Design review of the part built by this model. Coordinates are the model's own, in mm. A direction names the side the tool comes from. Round coordinates to 2 decimals unless told otherwise and drop trailing zeros. Order: outer loops, then holes, each group sorted by start corner. A loop starts at its lowest first (then second) coordinate and runs counter-clockwise, first axis right, second up. Notation, with made-up numbers: (75, -37) - (115, -37) arc R17 cw to (115, -19) - close; hole circle Ø11 at (-20, 64.25). An arc over 180 degrees is marked (long way). Use CSV: the item, a comma, the result in double quotes.
Autodesk Inventor part; units mm, degrees
ref_plane "YZ Plane" through (0, 0, 0) normal (1, 0, 0) x (0, 1, 0)
ref_plane "XZ Plane" through (0, 0, 0) normal (0, 1, 0) x (-1, 0, 0)
ref_plane "XY Plane" through (0, 0, 0) normal (0, 0, 1) x (1, 0, 0)
sketch "Sketch1" plane through (0, 0, 0) normal (1, 0, 0) x (0, 1, 0)
  line L0 (-25.5, 21) -> (25.5, 21)
  line L1 (25.5, 21) -> (25.5, -21)
  line L2 (25.5, -21) -> (-25.5, -21)
  line L3 (-25.5, -21) -> (-25.5, 21)
  line L4 (-25.5, 21) -> (25.5, -21) construction
  line L5 (25.5, 21) -> (-25.5, -21) construction
  circle A0 centre (15.5, 16) radius 1.6
  circle A1 centre (15.5, -16) radius 1.6
  circle A2 centre (-19.5, -16) radius 1.6
  circle A3 centre (-19.5, 16) radius 1.6
  line L6 (17.5, 0) -> (-17.5, 0) construction
  line L7 (17.5, 4) -> (-17.5, 4)
  line L8 (-17.5, -4) -> (17.5, -4)
  arc A4 (17.5, -4) -> (17.5, 4) centre (17.5, 0) ccw
  arc A5 (-17.5, 4) -> (-17.5, -4) centre (-17.5, 0) ccw
  point P0 (0, 0)
  point P1 (-9.5, -16)
  point P2 (0, 0)
  point P3 (15.5, -48)
  point P4 (-19.5, -35.5845)
  dimension "d0" = 42
  dimension "d1" = 51
  dimension "d2" = 5
  dimension "d3" = 10
  dimension "d5" = 35
  dimension "d6" = 5
  dimension "d7" = 3.2
  dimension "d8" = 3.2
  dimension "d9" = 3.2
  dimension "d10" = 3.2
  dimension "d15" = 0
  dimension "d16" = 0
  dimension "d17" = 32
  dimension "d18" = 0
  dimension "d19" = 0
  dimension "d20" = 8
  dimension "d21" = 8
  dimension "d22" = 8
  dimension "d31" = 32
extrude "Extrusion1" add sketch "Sketch1" along normal blind 5
fillet "Fillet1" radius 2 4 edges at (2.5, 25.5, 21) (2.5, -25.5, 21) (2.5, -25.5, -21) (2.5, 25.5, -21)
sketch "Sketch2" plane through (0, 25.5, 19) normal (0, 1, 0) x (1, 0, 0)
  line L0 (0, 38) -> (0, 0)
  point P0 (0, 19)
  point P1 (2.5, 19)
  dimension "d23" = 2.5
hole "Hole1" at (2.5, 25.5, 0) direction (0, -1, 0) diameter 3 depth 80.45
properties part number "2mm_double_for_pulley" material "アルミニウム 6061"
1) For faces 5 (the face through (2, 0, -4)), 6 (the face through (2.54, -24.9, 20.43)), list the 3-axis set-ups (+Z, -Z, +X, -X, +Y, -Y) from which the entire face can be reached by the end or side of a thin tool; tool diameter is ignored.
Data:
face 5,"+X, -X"
face 6,"+Z, +X, -X, -Y"
2) The part is to be moulded in two halves that separate along X. For faces 1 (the face through (2, 0, 4)), 2 (the face through (0, 0, 5)), 3 (the face through (2.43, 23.32, -1.5)), 4 (the face through (2.05, -23.38, 1.43)), say which applies: +X half, -X half, draft (parallel to the pull), parting line (faces both ways), or undercut.
Data:
face 1,"draft"
face 2,"-X half"
face 3,"undercut"
face 4,"undercut"
3) We need section C-C (y = 15.5). Give the boundary of the cut face in (x, z).
Data:
outline,"(0, -21) - (5, -21) - (5, -17.6) - (0, -17.6) - close; (0, -14.4) - (5, -14.4) - (5, -4) - (0, -4) - close; (0, 4) - (5, 4) - (5, 14.4) - (0, 14.4) - close; (0, 17.6) - (5, 17.6) - (5, 21) - (0, 21) - close"
4) We need section D-D (y = -14). Give the boundary of the cut face in (x, z), then the cut area to 3 significant figures.
Data:
outline,"(0, -21) - (5, -21) - (5, -4) - (0, -4) - close; (0, 4) - (5, 4) - (5, 21) - (0, 21) - close"
area,"170 mm2"
5) We need section A-A (x = 2.5). Give the boundary of the cut face in (y, z), then the cut area to 3 significant figures.
Data:
outline,"(-25.5, -19) arc R2 ccw to (-23.5, -21) - (23.5, -21) arc R2 ccw to (25.5, -19) - (25.5, -1.5) - (21.21, -1.5) arc R4 cw to (17.5, -4) - (-17.5, -4) arc R4 cw to (-21.21, -1.5) - (-25.5, -1.5) - close; (-25.5, 1.5) - (-21.21, 1.5) arc R4 cw to (-17.5, 4) - (17.5, 4) arc R4 cw to (21.21, 1.5) - (25.5, 1.5) - (25.5, 19) arc R2 ccw to (23.5, 21) - (-23.5, 21) arc R2 ccw to (-25.5, 19) - close; hole circle Ø3.2 at (-19.5, -16); hole circle Ø3.2 at (-19.5, 16); hole circle Ø3.2 at (15.5, -16); hole circle Ø3.2 at (15.5, 16)"
area,"1,750 mm2"
6) We need section B-B (z = 0). Give the boundary of the cut face in (x, y).
Data:
outline,"(0, -25.5) - (1, -25.5) - (1, -21.5) - (0, -21.5) - close; (0, 21.5) - (1, 21.5) - (1, 25.5) - (0, 25.5) - close; (4, -25.5) - (5, -25.5) - (5, -21.5) - (4, -21.5) - close; (4, 21.5) - (5, 21.5) - (5, 25.5) - (4, 25.5) - close"
7) To check wall thickness, follow L1, parallel to Z at x = 2.3, y = 15.5; L2, parallel to Z at x = 2.5, y = 23; L3, parallel to X at y = 24.3, z = 0. State the ranges of each line that lie inside material, in increasing order. Write a range as from..to.
Data:
L1,"z = -21..-17.6, -14.4..-4, 4..14.4, 17.6..21"
L2,"z = -21..-1.5, 1.5..21"
L3,"x = 0..1, 4..5"
